Part print with two shaded views. Sizes in mm from the minimum x, y, z corner. Coordinates: 2 decimals unless noted, no trailing zeros. Order: outer loops, then holes, each group sorted by start corner. A loop starts at its lowest first (then second) coordinate and runs counter-clockwise, first axis right, second up.
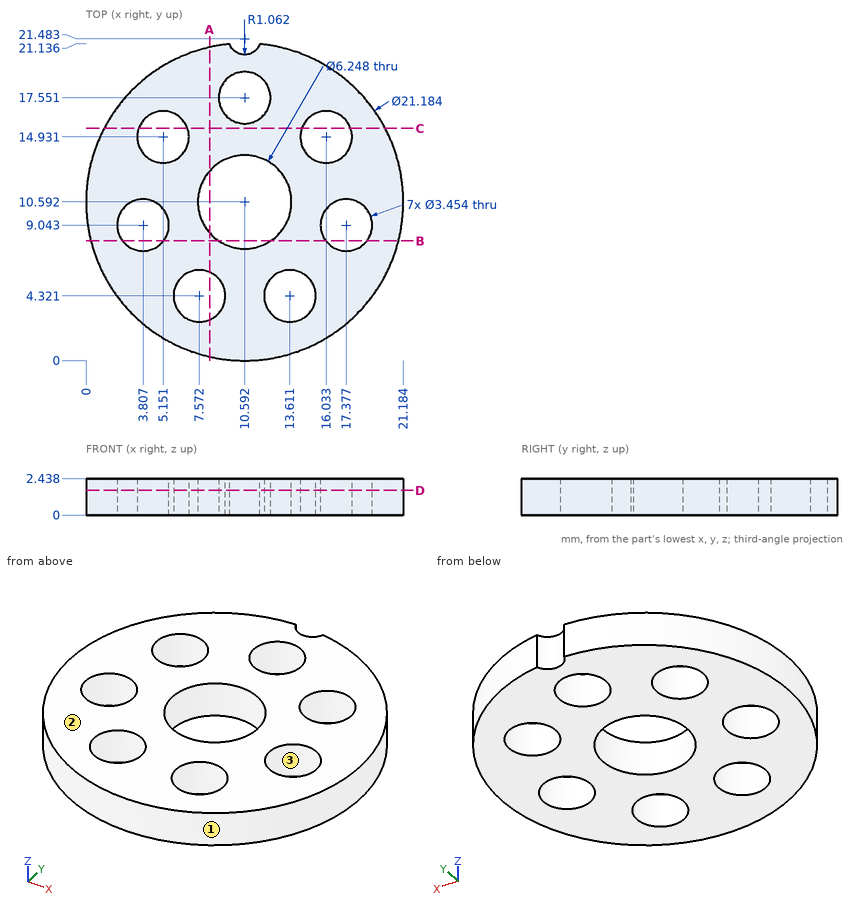
Q1. Wall check: line 1 along Y through (x, z) = (16.5, 1.75) (1 decimal); line 2 along Y through (x, z) = (3.75, 1.9) (1 decimal); line 3 along X through (y, z) = (14.5, 0.65) (1 decimal). Give the ranges that are in metal, low to high.
Results list:
line 1: y = 1.8 to 7.6, 10.5 to 13.3, 16.6 to 19.4
line 2: y = 2.5 to 7.3, 10.8 to 13.9, 15.9 to 18.7
line 3: x = 0.7 to 3.5, 6.8 to 14.4, 17.7 to 20.4
Q2. Pin check, flat tips, straight feed: pin 1 Ø2 at (x, y) = (10.59, 17.55) entering from +Z (3 decimals); pin 2 Ø3 at (x, y) = (10.5, 14) entering from -Z; pin 3 Ø1 at (y, z) = (12, 1) entering from +X (1 decimal). Stop position of each tip, or through.
Results list:
pin 1: passes through
pin 2: stops at z = 0
pin 3: stops at x = 21.1
Q3. Cut at C-C on y = 15.5. Write the cut outline in (x, z) (1 decimal).
Results list:
outline: (1.2, 0) - (3.5, 0) - (3.5, 2.4) - (1.2, 2.4) - close; (6.8, 0) - (14.4, 0) - (14.4, 2.4) - (6.8, 2.4) - close; (17.7, 0) - (20, 0) - (20, 2.4) - (17.7, 2.4) - close
Q4. Mould opens along Y. For the marked faces 1, 2 and 3 say: pulls with the +Y half, pulls with the -Y half, needs draft (parallel to the pull), parting line crosses it, or undercut.
Results list:
face 1: parting line crosses it
face 2: needs draft
face 3: undercut
Q5. Cut at A-A on x = 8.25. Write the cut outline in (y, z).
Results list:
outline: (0.26, 0) - (2.73, 0) - (2.73, 2.44) - (0.26, 2.44) - close; (5.91, 0) - (8.52, 0) - (8.52, 2.44) - (5.91, 2.44) - close; (12.66, 0) - (20.92, 0) - (20.92, 2.44) - (12.66, 2.44) - close
Q6. Cut at B-B on y = 8. Write the cut outline in (x, z).
Results list:
outline: (0.32, 0) - (2.43, 0) - (2.43, 2.44) - (0.32, 2.44) - close; (5.18, 0) - (8.85, 0) - (8.85, 2.44) - (5.18, 2.44) - close; (12.34, 0) - (16, 0) - (16, 2.44) - (12.34, 2.44) - close; (18.75, 0) - (20.86, 0) - (20.86, 2.44) - (18.75, 2.44) - close
Q7. Cut at D-D on z = 1.65. Count the separate pieces of the cut face and the enclosed holes in it, and give its area (3 significant figures).
Results list:
separate pieces: 1
enclosed holes: 8
area: 255 mm2
